The listing builds one solid part. Answer for the finished solid, in the listing's coordinates (mm). A direction names the side the tool comes from. Give positions to 0.01 mm unless a question says otherwise; leave off trailing zeros. Write each loop counter-clockwise with the first axis right and the second up, starting at its lowest first coordinate (ties: lowest second). Pieces come first, ordered by that corner, then holes. Notation, with made-up numbers: (-27, -30) - (0, -30) arc R16 ccw to (0, -22) - close; hole circle Ø11 at (65.5, 12). An arc over 180 degrees is marked (long way). One line per item, written item: value. Start each with the question number.
from build123d import *

# Parameters (mm, degrees)
F0_W     = 146.05
F0_H     = 79.375
F5_W     = 146.05
F5_H     = 12.7
F6_DEPTH = 9.525


with BuildPart() as f3:
    # F0 (on Top) → F3 section 0
    with BuildSketch(Plane.XY, mode=Mode.PRIVATE) as f3_s0:
        Rectangle(F0_W, F0_H)
    loft([f3_s0.sketch, Vertex(0, 0, 38.1)])

    # F5 (on offset) → F6 (join)
    with BuildSketch(Plane.XY):
        with Locations((0, -30.1625)):
            Rectangle(F5_W, F5_H)
    extrude(amount=-F6_DEPTH)


solid = f3.part
Item 1: For faces 1 (the flat face through (0, -38, 0)), 2 (the flat face through (-44.12, 0.56, 15.08)), 3 (the flat face through (-1, 8, 0)), determine the directions among +Z, -Z, +X, -X, +Y, -Y from which every point of the face is accessible in a straight line to the end or side of a thin tool.
Item 2: Find section B-B on z = 34.5. Determine the outline of the cut face in (x, y).
Item 3: Find section A-A on x = 38. Determine the outline of the cut face in (y, z) (1 decimal).
Item 4: Each of these flat-tipped pins is pushed along its axis until it touches: pin 1 Ø6 at (y, z) = (-30, 9.5) entering from +X; pin 2 Ø5 at (x, y) = (56, 26.5) entering from -Z; pin 3 Ø4 at (y, z) = (22, 13) entering from +X. Where does it stop, or does it pass through?
Item 5: Straight lines are drawn through the part: line 1 along Y through (x, z) = (27.5, -1); line 2 along Z through (x, y) = (26, 31); line 3 along Z through (x, y) = (51, -17). For each, find the intervals that lie inside material, in ascending order.
Item 6: Find section C-C on y = -35. Determine the outline of the cut face in (x, z) (3 decimals), plus the area to 3 significant figures.
Item 7: Find section D-D on x = -24. Determine the outline of the cut face in (y, z) (1 decimal).
Values:
1. face 1: -Z, +X, -X, -Y
1. face 2: +Z, -X, +Y, -Y
1. face 3: -Z, +X, -X, +Y
2. outline: (-6.9, -3.75) - (6.9, -3.75) - (6.9, 3.75) - (-6.9, 3.75) - close
3. outline: (-39.7, 0) - (-36.5, 0) - (-36.5, -9.5) - (-23.8, -9.5) - (-23.8, 0) - (39.7, 0) - (20.7, 18.3) - (-20.7, 18.3) - close
4. pin 1: x = 60.57
4. pin 2: z = 0
4. pin 3: x = 51.94
5. line 1: -36.51 to -23.81
5. line 2: 0 to 8.34
5. line 3: 0 to 11.49
6. outline: (-73.025, -9.525) - (73.025, -9.525) - (73.025, 0) - (64.4, 4.5) - (-64.4, 4.5) - (-73.025, 0) - close
6. area: 2,010 mm^2
7. outline: (-39.7, 0) - (-36.5, 0) - (-36.5, -9.5) - (-23.8, -9.5) - (-23.8, 0) - (39.7, 0) - (13, 25.6) - (-13, 25.6) - close
